For this review, take the finished solid that the model builds, in its own axes (mm). Face numbers are marked on the shaded views. A direction names the side the tool comes from. Coordinates: 2 decimals unless noted, no trailing zeros. Loops run counter-clockwise (first coordinate to the right, second up) from the corner with the lowest first, then second, coordinate; pieces in that order, holes last. Notation, with made-up numbers: M 12.25,88 L 53.25,88 A32 cw 53.25,124 Z; hole C 2.5,76.25 d2. An arc over 180 degrees is marked long. Put each result on its own line as item: value.
```python
from build123d import *

# Parameters (mm, degrees)
F2_W     = 50
F2_H     = 50
F3_DEPTH = 30
F4_T     = -2
F5_R     = 4


with BuildPart() as f3:
    # F2 (on Top) → F3 (new body)
    with BuildSketch(Plane.XY):
        Rectangle(F2_W, F2_H)
    extrude(amount=F3_DEPTH)

    # F4
    f4_openings = [f3.faces().sort_by_distance(p)[0] for p in [
        (0, 0, 30),
    ]]
    offset(amount=F4_T, openings=f4_openings)

    # F5
    f5_edges = [f3.edges().sort_by_distance(p)[0] for p in [
        (0, 23, 2),
        (-23, 0, 2),
        (23, 0, 2),
        (0, -23, 2),
    ]]
    fillet(f5_edges, radius=F5_R)


solid = f3.part
```
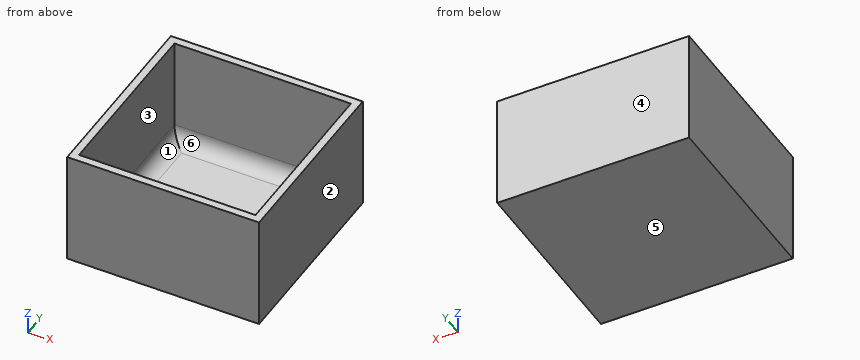
(1) For pin 1 (5 mm diameter, centred on x = 15.5, y = -0.5, fed in from +Z), flat-tipped, find the tip position at first contact; note if it passes through.
Determined:
pin 1: stops at z = 2
(2) Tool access review of the marked faces 5 and 6: name each direction out of +Z, -Z, +X, -X, +Y, -Y from which nothing blocks a thin tool from reaching the whole face with its end or side.
Determined:
face 5: -Z, +X, -X, +Y, -Y
face 6: +Z
(3) Add section C-C (z = 21.75). Write out the cut boundary in (x, y).
Determined:
outline: M -25,-25 L 25,-25 L 25,25 L -25,25 Z; hole M -23,-23 L 23,-23 L 23,23 L -23,23 Z
(4) Add section D-D (z = 4.5). Write out the cut boundary in (x, y).
Determined:
outline: M -25,-25 L 25,-25 L 25,25 L -25,25 Z; hole M -22.71,-22.71 L 22.71,-22.71 L 22.71,22.71 L -22.71,22.71 Z
(5) Wall thickness on line 1 along X through (y, z) = (-5.5, 25); line 2 along Z through (x, y) = (-19, -1.5): over which ranges is each line inside the solid? List them lowest first. Write a range as [from, to].
Determined:
line 1: x = [-25, -23], [23, 25]
line 2: z = [0, 2]
(6) Draft analysis for pull direction Y (two halves, no side actions). For the marked faces 1, 2, 3 and 4, state which applies: +Y half, -Y half, draft (parallel to the pull), parting line (faces both ways), or undercut.
Determined:
face 1: undercut
face 2: draft
face 3: undercut
face 4: +Y half
(7) Add section A-A (y = 11). Write out the cut boundary in (x, z).
Determined:
outline: M -25,0 L 25,0 L 25,30 L 23,30 L 23,6 A4 cw 19,2 L -19,2 A4 cw -23,6 L -23,30 L -25,30 Z
